Part print with two shaded views. Sizes in mm from the minimum x, y, z corner. Coordinates: 2 decimals unless noted, no trailing zeros. Order: outer loops, then holes, each group sorted by start corner. A loop starts at its lowest first (then second) coordinate and runs counter-clockwise, first axis right, second up. Notation, with made-up numbers: (25, 15.5) - (37, 15.5) arc R21 ccw to (37, 34.5) - close; hole circle Ø4 at (18.25, 76.25). An arc over 180 degrees is marked (long way). Write each question's results on one line, items separated by ' | '. Start each with the question number.
Q1. Pin check, flat tips, straight feed: P1, Ø4, axis at x = 6, y = 3, coming from the -Z side; P2, Ø3, axis at x = 8, y = 3, coming from the -Z side. Stop position of each tip, or through.
Q2. Band-saw the part on C-C, the plane y = 1.75. Write the cut outline in (x, z) (1 decimal).
Q3. Band-saw the part on A-A, the plane x = 7.75. Write the cut outline in (y, z) (1 decimal).
Q4. Wall check: probe 1 along Y at (x, z) = (2.5, 11); probe 2 along Z at (x, y) = (2.5, 5) (1 decimal); probe 3 along Z at (x, y) = (9, 5.5) (1 decimal). Give the ranges that are in metal, low to high.
Q5. Band-saw the part on B-B, the plane z = 2.5. Write the cut outline in (x, y), then the cut area to 3 significant figures.
Q6. Pull direction Y, two halves, no side cores. Call the marked faces 1, 2, 3 and 4: released by +Y, released by -Y, zero draft, split by the parting line, or undercut.
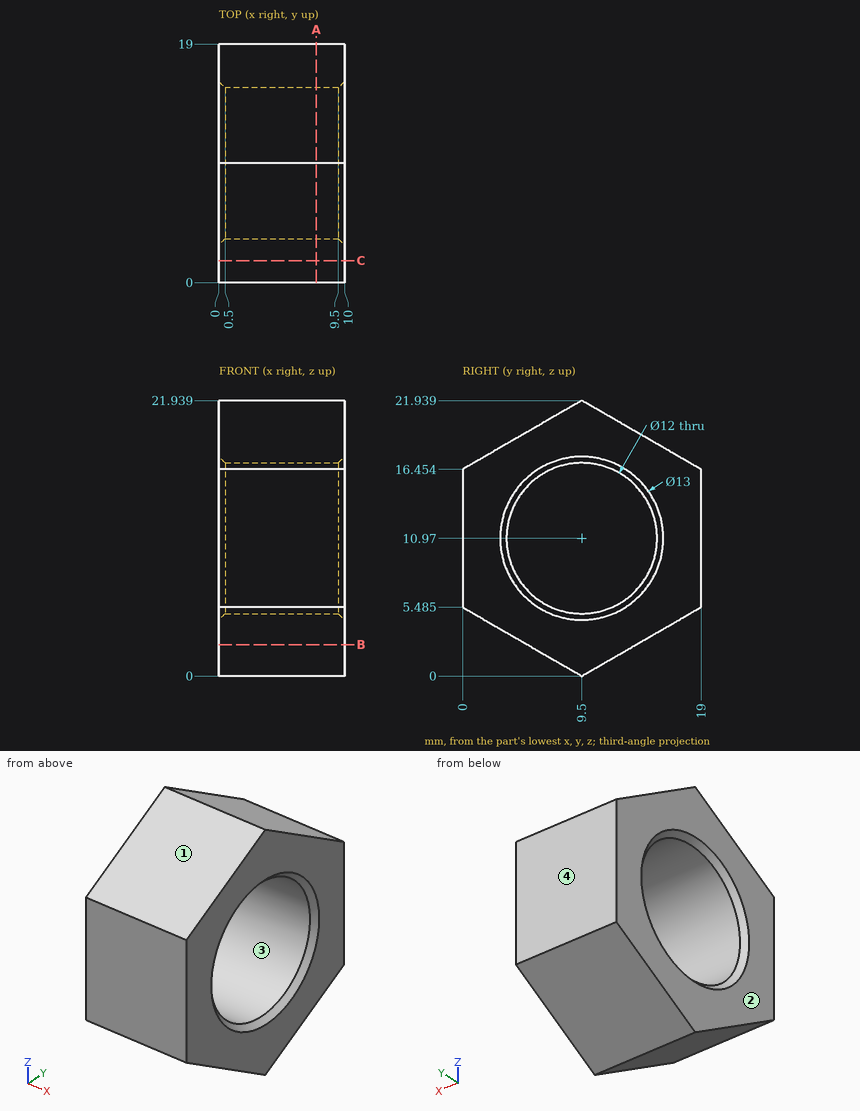
Results below:
1) P1: stops at z = 2.6 | P2: stops at z = 2.89
2) outline: (0, 4.5) - (10, 4.5) - (10, 17.5) - (0, 17.5) - close
3) outline: (0, 5.5) - (9.5, 0) - (19, 5.5) - (19, 16.5) - (9.5, 21.9) - (0, 16.5) - close; hole circle Ø12 at (9.5, 11)
4) probe 1: y = 0 to 3.5, 15.5 to 19 | probe 2: z = 2.6 to 7, 14.9 to 19.3 | probe 3: z = 2.3 to 6.5, 15.4 to 19.6
5) outline: (0, 5.17) - (10, 5.17) - (10, 13.83) - (0, 13.83) - close | area: 86.6 mm²
6) face 1: released by -Y | face 2: zero draft | face 3: undercut | face 4: released by +Y
